Can you work these out from the model? Positions are in its coordinate system, mm. A direction names the side the tool comes from. Give positions to 0.01 mm unless a question says otherwise; leave off trailing zeros. Write each loop counter-clockwise with the first axis right and the second up, starting at its lowest first coordinate (ties: lowest second). Pieces come first, ordered by that corner, then holes. Notation, with made-up numbers: (86.5, 75.25) -> (120.5, 75.25) arc R19 cw to (120.5, 82.25) -> close; hole circle Ø8 at (77.5, 30.5). An arc over 180 degrees is marked (long way). Answer as CSV lines item,"result". Start each with the question number.
1. I need wall thicknesses on line 1 (Z direction, x = 0, y = -3.25); line 2 (Z direction, x = -0.75, y = 4.25); line 3 (X direction, y = -7, z = 17.75). Which ranges of each line are inside material? Lowest first, please. Write a range as [from, to].
2. I'm going to push flat-ended pins straight in: P1, Ø4, axis at y = -7, z = 15, coming from the -X side; P2, Ø2, axis at y = 1.5, z = 12, coming from the +X side; P3, Ø1, axis at x = -8, y = -7, coming from the +Z side. Where does each tip first touch, or does it pass through?
3. On a 3-axis mill with a long thin cutter (end or side, diameter ignored), from which of +Z, -Z, +X, -X, +Y, -Y can I reach the whole of each face in a straight line? I mean faces 1 (the face through (-5.8, 0, 7.7)), 2 (the face through (-8.61, -8.5, 15.07)). Say none if no direction works.
4. If we mould it in two halves opening along Z, with no side actions, what happens to faces 3 (the face through (8, -10, 18)), 4 (the face through (7.62, -2.39, 11.84)), 5 (the face through (-2.38, 0.51, 4.26))? For each: pulls with the +Z half, pulls with the -Z half, needs draft (parallel to the pull), parting line crosses it, or undercut.
5. If we section it at C-C on x = 0: Write out the boundary of the cut face in (y, z).
6. If we section it at B-B on y = -6.5: Write out the boundary of the cut face in (x, z).
7. If we section it at A-A on z = 15: Write out the boundary of the cut face in (x, y), plus the area to 3 significant figures.
8. If we section it at D-D on y = -3.75: Write out the boundary of the cut face in (x, z).
```python
from build123d import *

# Parameters (mm, degrees)
SKETCH013_R      = 11
SKETCH013_R_2    = 8.25
PAD007_DEPTH     = 15
SKETCH014_R      = 11.25
SKETCH014_R_2    = 9.25
POCKET006_DEPTH  = 12
CHAMFER006_SIZE2 = 1.5
CHAMFER006_SIZE  = 4
SKETCH015_R      = 1.25
HOLE_DEPTH       = 25
CHAMFER008_SIZE2 = 1
CHAMFER008_SIZE  = 4
SKETCH054_R      = 1.5
POCKET021_DEPTH  = 20


with BuildPart() as part:
    # Sketch013 → Pad007 (new body)
    with BuildSketch(Plane.XZ.offset(-10)):
        with Locations((0, 15)):
            Circle(SKETCH013_R)
        with Locations((0, 15)):
            Circle(SKETCH013_R_2, mode=Mode.SUBTRACT)
    extrude(amount=PAD007_DEPTH)

    # Sketch014 → Pocket006 (cut)
    with BuildSketch(Plane.XZ.offset(7)):
        with Locations((0.134772, 15)):
            Circle(SKETCH014_R)
        with Locations((0.134772, 15)):
            Circle(SKETCH014_R_2, mode=Mode.SUBTRACT)
    extrude(amount=-POCKET006_DEPTH, mode=Mode.SUBTRACT)

    # Chamfer006
    chamfer006_edges = [part.edges().sort_by_distance(p)[0] for p in [
        (-11, 10, 15),
    ]]
    chamfer006_side = part.faces().sort_by_distance((-11, 7.5, 15))[0]
    chamfer(chamfer006_edges, length=CHAMFER006_SIZE, length2=CHAMFER006_SIZE2, reference=chamfer006_side)

    # Sketch015 → Hole (cut)
    with BuildSketch(Plane(origin=(0, 4, 5), x_dir=(1, 0, 0), z_dir=(0, 0, 1))):
        with Locations((0.028156, -7.033275)):
            Circle(SKETCH015_R)
    extrude(amount=-HOLE_DEPTH, mode=Mode.SUBTRACT)

    # Chamfer008
    chamfer008_edges = [part.edges().sort_by_distance(p)[0] for p in [
        (-9.5, 10, 15),
    ]]
    chamfer008_side = part.faces().sort_by_distance((-10.25, 8, 15))[0]
    chamfer(chamfer008_edges, length=CHAMFER008_SIZE, length2=CHAMFER008_SIZE2, reference=chamfer008_side)

    # Sketch054 → Pocket021 (cut)
    with BuildSketch(Plane.YZ.offset(10)):
        with Locations((-2, 15)):
            Circle(SKETCH054_R)
    extrude(amount=-POCKET021_DEPTH, mode=Mode.SUBTRACT)


with BuildPart() as part_1:
    # Body006 placement: moved
    add(part.part.moved(Location((0, -5, 0))))


solid = part_1.part
```
Computed values:
1,line 1,"z = [5.75, 6.75], [23.25, 24.25]"
1,line 2,"z = [6.05, 6.78], [23.22, 23.95]"
1,line 3,"x = [-8.7, -7.78], [7.78, 8.97]"
2,P1,"stops at x = -9.12"
2,P2,"stops at x = 10.79"
2,P3,"stops at z = 20.22"
3,face 1,"-Y"
3,face 2,"+X, -X"
4,face 3,"needs draft"
4,face 4,"undercut"
4,face 5,"parting line crosses it"
5,outline,"(-10, 5.75) -> (0, 5.75) -> (0, 4) -> (1, 4) -> (1.25, 4.1) -> (5, 6.5) -> (5, 6.75) -> (-10, 6.75) -> close; (-10, 23.25) -> (5, 23.25) -> (5, 23.5) -> (1.25, 25.9) -> (1, 26) -> (0, 26) -> (0, 24.25) -> (-10, 24.25) -> close"
6,outline,"(-9.01, 13.59) arc R9.25 ccw to (9.28, 13.59) -> (8.13, 13.59) arc R8.25 cw to (-8.13, 13.59) -> close; (-9.01, 16.41) -> (-8.13, 16.41) arc R8.25 cw to (8.13, 16.41) -> (9.28, 16.41) arc R9.25 ccw to start"
7,outline,"(-11, 0) -> (-9.12, 0) -> (-9.12, -5.5) -> (-8.25, -5.5) -> (-8.25, 5) -> (-8.5, 5) -> (-10.9, 1.25) -> (-11, 1) -> close; (-9.12, -10) -> (-8.25, -10) -> (-8.25, -8.5) -> (-9.12, -8.5) -> close; (8.25, -10) -> (9.38, -10) -> (9.38, -8.5) -> (8.25, -8.5) -> close; (8.25, -5.5) -> (9.38, -5.5) -> (9.38, 0) -> (11, 0) -> (11, 1) -> (10.9, 1.25) -> (8.5, 5) -> (8.25, 5) -> close"
7,area,"31.8 mm2"
8,outline,"circle Ø18.5 at (0.13, 15); hole circle Ø16.5 at (0, 15)"
